Read the model definition and answer for the solid it produces. Units are mm, in the model's axes. A direction names the side the tool comes from. Give positions to 0.01 mm unless a question says otherwise; leave off trailing zeros. Loops run counter-clockwise (first coordinate to the right, second up) from the corner with the lowest first, then second, coordinate; pieces in that order, holes last. Notation, with made-up numbers: (50, 49.25) -> (87, 49.25) arc R29 cw to (87, 71.25) -> close; hole circle Ø9 at (67, -29.5). An arc over 180 degrees is marked (long way). Write each question's results on one line, items separated by ' | '. Start each with the question number.
Item 1: Section C-C on z = -21.5 is taken. Write down the section's boundary in (x, y).
Item 2: Which of the six approach directions +Z, -Z, +X, -X, +Y, -Y give full straight-line access (tool end or side, diameter ignored) to faces 1 (the flat face through (-10, 0, -15)), 2 (the flat face through (8.2, 72.3, 60)), 3 (the flat face through (0, 5, -62))?
Item 3: Each of these flat-tipped pins is pushed along its axis until it touches: P1, Ø1.5, axis at x = 3, y = 7, coming from the -Z side; P2, Ø8, axis at x = 37, z = 18, coming from the -Y side; P3, Ø10, axis at x = -93.5, y = -7.5, coming from the +Z side. Where does it stop, or does it pass through?
Item 4: Section B-B on z = -47 is taken. Write down the section's boundary in (x, y) (3 decimals).
Item 5: Find the intervals of material crossed by line 1 (Z direction, x = 45.5, y = 38); line 2 (Z direction, x = -87.5, y = -39); line 3 (Y direction, x = 5, z = -30) (3 decimals), in increasing order.
```python
from build123d import *

# Parameters (mm, degrees)
SCHIZZO1_R                    = 125
ESTRUSIONE_ESTRUSIONE1_DEPTH  = 60
SCHIZZO2_R                    = 62.5
ESTRUSIONE_ESTRUSIONE2_DEPTH  = 10
SCHIZZO3_R                    = 22.5
ESTRUSIONE_ESTRUSIONE3_DEPTH  = 15
SCHIZZO4_R                    = 8
ESTRUSIONE_ESTRUSIONE4_DEPTH  = 70
RACCORDO1_R                   = 10
RACCORDO2_R                   = 28
TAGLIO_ESTRUSIONE1_DEPTH      = 236.887520145
TAGLIO_ESTRUSIONE1_DEPTH_BACK = 45


with BuildPart() as part:
    # Schizzo1 → Estrusione-Estrusione1 (new body)
    with BuildSketch(Plane.XY):
        with Locations((1.463125693, 0)):
            Circle(SCHIZZO1_R)
    extrude(amount=ESTRUSIONE_ESTRUSIONE1_DEPTH)

    # Schizzo2 → Estrusione-Estrusione2 (add)
    with BuildSketch(Plane.XY.offset(60)):
        Circle(SCHIZZO2_R)
    extrude(amount=ESTRUSIONE_ESTRUSIONE2_DEPTH)

    # Schizzo3 → Estrusione-Estrusione3 (add)
    with BuildSketch(Plane(origin=(0, 0, 0), x_dir=(-1, 0, 0), z_dir=(0, 0, -1))):
        Circle(SCHIZZO3_R)
    extrude(amount=ESTRUSIONE_ESTRUSIONE3_DEPTH)

    # Schizzo4 → Estrusione-Estrusione4 (add)
    with BuildSketch(Plane(origin=(0, 0, -15), x_dir=(-1, 0, 0), z_dir=(0, 0, -1))):
        Circle(SCHIZZO4_R)
    extrude(amount=ESTRUSIONE_ESTRUSIONE4_DEPTH)

    # Raccordo1
    raccordo1_edges = [part.edges().sort_by_distance(p)[0] for p in [
        (-62.5, 0, 60),
        (22.5, 0, 0),
    ]]
    fillet(raccordo1_edges, radius=RACCORDO1_R - 0.0001)  # a hair under: the kernel refuses the full size

    # Raccordo2
    raccordo2_edges = [part.edges().sort_by_distance(p)[0] for p in [
        (-123.536874307, 0, 0),
        (-123.536874307, 0, 60),
    ]]
    fillet(raccordo2_edges, radius=RACCORDO2_R)

    # Schizzo5 → Taglio-Estrusione1 (cut, two sides: drawn at the far end of the back side and taken through both)
    with BuildSketch(Plane(origin=(0, 0, -85), x_dir=(-1, 0, 0), z_dir=(0, 0, -1)).offset(-TAGLIO_ESTRUSIONE1_DEPTH_BACK)):
        Polygon((-387.790129005, 5), (-6.244997998, 5), (6.244997998, 5), (387.790129005, 5), (387.790129005, 768.090262014), (-387.790129005, 768.090262014), align=None)
    extrude(amount=TAGLIO_ESTRUSIONE1_DEPTH + TAGLIO_ESTRUSIONE1_DEPTH_BACK, mode=Mode.SUBTRACT)


solid = part.part
```
Findings:
1) outline: circle Ø16 at (0, 0)
2) face 1: -Z | face 2: +Z | face 3: -Z, +X, -X, +Y
3) P1: z = -40 | P2: y = -119.68 | P3: z = 60
4) outline: (-6.245, 5) arc R8 ccw (long way) to (6.245, 5) -> close
5) line 1: 0 to 70 | line 2: 0 to 60 | line 3: -6.245 to 6.245
